Design review of the part shown in the three views and the two pictorial views. Dimensions are in mm from the part's minimum x, y and z. A direction names the side the tool comes from. Coordinates: 2 decimals unless noted, no trailing zeros. Write each loop counter-clockwise with the first axis right and the second up, starting at its lowest first coordinate (ties: lowest second). Pieces come first, ordered by that corner, then holes. Notation, with made-up numbers: M -37.75,89 L 9.25,89 A19 ccw 9.25,113 Z; hole C 88,59 d5. An arc over 180 degrees is marked long. One line per question, with ' | ' between items.
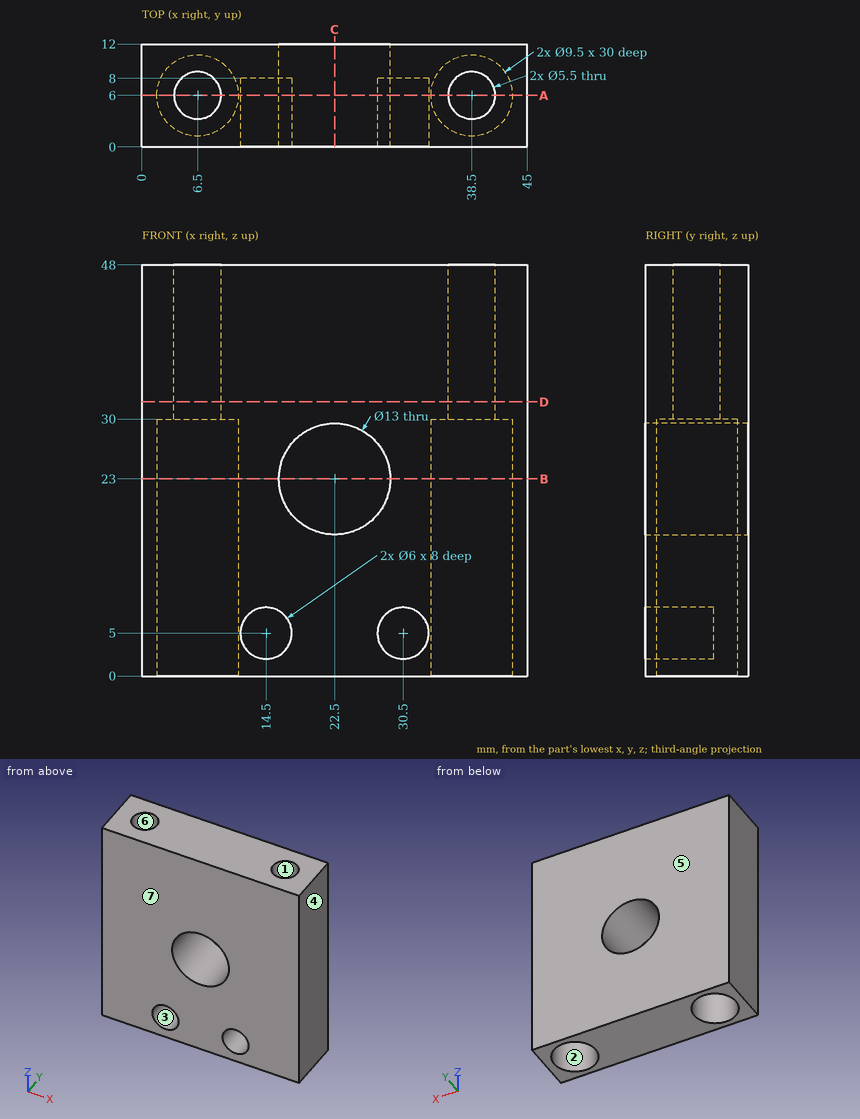
1. Clearance check with a flat-ended pin moving along its axis: P1, Ø7, axis at x = 6.5, y = 6, coming from the -Z side. State where the tip first meets the part, or that it passes through.
Computed values:
P1: stops at z = 30
2. For line 1 along X through (y, z) = (8.75, 27.5); line 2 along X through (y, z) = (5.75, 40); line 3 along Y through (x, z) = (38.5, 37.5), list the stretches that pass through material, from the lowest coordinate up.
Computed values:
line 1: x = 0 to 2.63, 10.37 to 17.81, 27.19 to 34.63, 42.37 to 45 | line 2: x = 0 to 3.76, 9.24 to 35.76, 41.24 to 45 | line 3: y = 0 to 3.25, 8.75 to 12
3. Take a section at D-D on z = 32. State the section outline as (x, y) points.
Computed values:
outline: M 0,0 L 45,0 L 45,12 L 0,12 Z; hole C 6.5,6 d5.5; hole C 38.5,6 d5.5
4. Take a section at B-B on z = 23. State the section outline as (x, y) points.
Computed values:
outline: M 0,0 L 16,0 L 16,12 L 0,12 Z; M 29,0 L 45,0 L 45,12 L 29,12 Z; hole C 6.5,6 d9.5; hole C 38.5,6 d9.5
5. Take a section at C-C on x = 22.5. State the section outline as (y, z) points.
Computed values:
outline: M 0,0 L 12,0 L 12,16.5 L 0,16.5 Z; M 0,29.5 L 12,29.5 L 12,48 L 0,48 Z
6. Take a section at A-A on y = 6. State the section outline as (x, z) points, plus the area to 3 significant figures.
Computed values:
outline: M 0,0 L 1.75,0 L 1.75,30 L 3.75,30 L 3.75,48 L 0,48 Z; M 9.25,30 L 11.25,30 L 11.25,0 L 33.75,0 L 33.75,30 L 35.75,30 L 35.75,48 L 9.25,48 Z; M 41.25,30 L 43.25,30 L 43.25,0 L 45,0 L 45,48 L 41.25,48 Z; hole C 14.5,5 d6; hole C 22.5,23 d13; hole C 30.5,5 d6 | area: 1,200 mm2
7. Machinability: for the marked faces 1, 2 and 3, which of the approach directions +Z, -Z, +X, -X, +Y, -Y give a long, thin tool a straight path to every point of the face, cutting with its end or side? Answer none if there is none.
Computed values:
face 1: +Z, -Z | face 2: -Z | face 3: -Y
8. Draft analysis for pull direction Y (two halves, no side actions). For the marked faces 4, 5, 6 and 7, state which applies: pulls with the +Y half, pulls with the -Y half, needs draft (parallel to the pull), parting line crosses it, or undercut.
Computed values:
face 4: needs draft | face 5: pulls with the +Y half | face 6: undercut | face 7: pulls with the -Y half
